from build123d import *

# Parameters (mm, degrees)
SKETCH_1_R               = 9
SKETCH_1_R_2             = 1.5
EXTRUDE_1_DEPTH          = 5
EXTRUDE_START            = -5
EXTRUDE_2_DEPTH          = 5
PATTERN_CIRCULAR_1_COUNT = 10


with BuildPart() as part:
    # 草图1 → 凸台-拉伸1 (new body)
    with BuildSketch(Plane(origin=(0, 0, 0), x_dir=(1, 0, 0), z_dir=(0, 1, 0))):
        with Locations(Location((0, 0, 0), (0, 0, 270))):
            Circle(SKETCH_1_R)
        with Locations(Location((0, 0, 0), (0, 0, 270))):
            Circle(SKETCH_1_R_2, mode=Mode.SUBTRACT)
    extrude(amount=EXTRUDE_1_DEPTH)

    # 草图2 → 凸台-拉伸2 (add)
    with BuildSketch(Plane(origin=(0, 5, 0), x_dir=(1, 0, 0), z_dir=(0, 1, 0)).offset(EXTRUDE_START)):
        with BuildLine():
            Line((1.5, 8.874119675), (1, 10.5))
            Line((1, 10.5), (-1, 10.5))
            Line((-1, 10.5), (-1.5, 8.874119675))
            ThreePointArc((-1.5, 8.874119675), (0, 9), (1.5, 8.874119675))
        make_face()
    extrude_2 = extrude(amount=EXTRUDE_2_DEPTH)

    # 阵列(圆周)1: 凸台-拉伸2 ×10 about axis
    pattern_circular_1_axis = Axis((0, 0, 0), (0, 1, 0))
    for i in range(1, PATTERN_CIRCULAR_1_COUNT):
        add(extrude_2.rotate(pattern_circular_1_axis, i * 360 / PATTERN_CIRCULAR_1_COUNT))


solid = part.part
Design review of the part built by this model. Coordinates are the model's own, in mm. A direction names the side the tool comes from. Coordinates: 2 decimals unless noted, no trailing zeros. Write each loop counter-clockwise with the first axis right and the second up, starting at its lowest first coordinate (ties: lowest second). Pieces come first, ordered by that corner, then holes. Notation, with made-up numbers: (70, -3.5) - (86, -3.5) arc R23 cw to (86, 16.5) - close; hole circle Ø10 at (-11.5, 70). An arc over 180 degrees is marked (long way). One line per item, written item: value.
1) Insertion check: pin 1 (5 mm diameter, centred on x = 0, z = 0, fed in from +Y); pin 2 (3 mm diameter, centred on y = 3.5, z = 7, fed in from +X); pin 3 (1 mm diameter, centred on y = 3, z = -6.5, fed in from -X); pin 4 (3 mm diameter, centred on y = 1.5, z = -5.5, fed in from -X). Each pin has a flat end and moves straight along its axis. Give the tip position at first contact, or say it passes through.
Answer sheet:
pin 1: stops at y = 5
pin 2: stops at x = 7.12
pin 3: stops at x = -6.71
pin 4: stops at x = -9.74
2) Add section B-B (z = 0). State the section outline as (x, y) points, plus the area to 3 significant figures.
Answer sheet:
outline: (-9, 0) - (-1.5, 0) - (-1.5, 5) - (-9, 5) - close; (1.5, 0) - (9, 0) - (9, 5) - (1.5, 5) - close
area: 75.0 mm2
3) Add section A-A (x = 0). State the section outline as (y, z) points, plus the area to 3 significant figures.
Answer sheet:
outline: (0, -10.5) - (5, -10.5) - (5, -1.5) - (0, -1.5) - close; (0, 1.5) - (5, 1.5) - (5, 10.5) - (0, 10.5) - close
area: 90.0 mm2
4) Mouldability with a two-part tool opening along Z and no side actions: class faces 4 (the face through (2.764, 2.465, 8.565)), 5 (the face through (-7.29, 2.46, 5.28)), 6 (the face through (-2, 5, 0)) as +Z half, -Z half, draft (parallel to the pull), parting line (faces both ways), or undercut.
Answer sheet:
face 4: +Z half
face 5: undercut
face 6: draft
5) To check wall thickness, follow probe 1 along X at (y, z) = (4.65, -1.25); probe 2 along X at (y, z) = (4.2, 9); probe 3 along Z at (x, y) = (3.25, 2.7). State the ranges of each line that lie inside material, in increasing order.
Answer sheet:
probe 1: x = -8.91 to -0.83, 0.83 to 8.91
probe 2: x = -5.48 to -5.25, -1.46 to 1.46, 5.25 to 5.48
probe 3: z = -8.39 to 8.39
6) Add section D-D (x = 4.5). State the section outline as (y, z) points, plus the area to 3 significant figures.
Answer sheet:
outline: (0, -8.43) - (5, -8.43) - (5, 8.43) - (0, 8.43) - close
area: 84.3 mm2
7) For faces 1 (the face through (4.692, 2.465, -8.579)), 2 (the face through (9.61, 2.46, 1.81)), 3 (the face through (-6.7, 2.46, 7.09)), list the 3-axis set-ups (+Z, -Z, +X, -X, +Y, -Y) from which the entire face can be reached by the end or side of a thin tool; tool diameter is ignored.
Answer sheet:
face 1: -Z, +Y, -Y
face 2: +X, +Y, -Y
face 3: -X, +Y, -Y
8) Add section C-C (z = -6.75). State the section outline as (x, y) points.
Answer sheet:
outline: (-6.58, 0) - (6.58, 0) - (6.58, 5) - (-6.58, 5) - close
